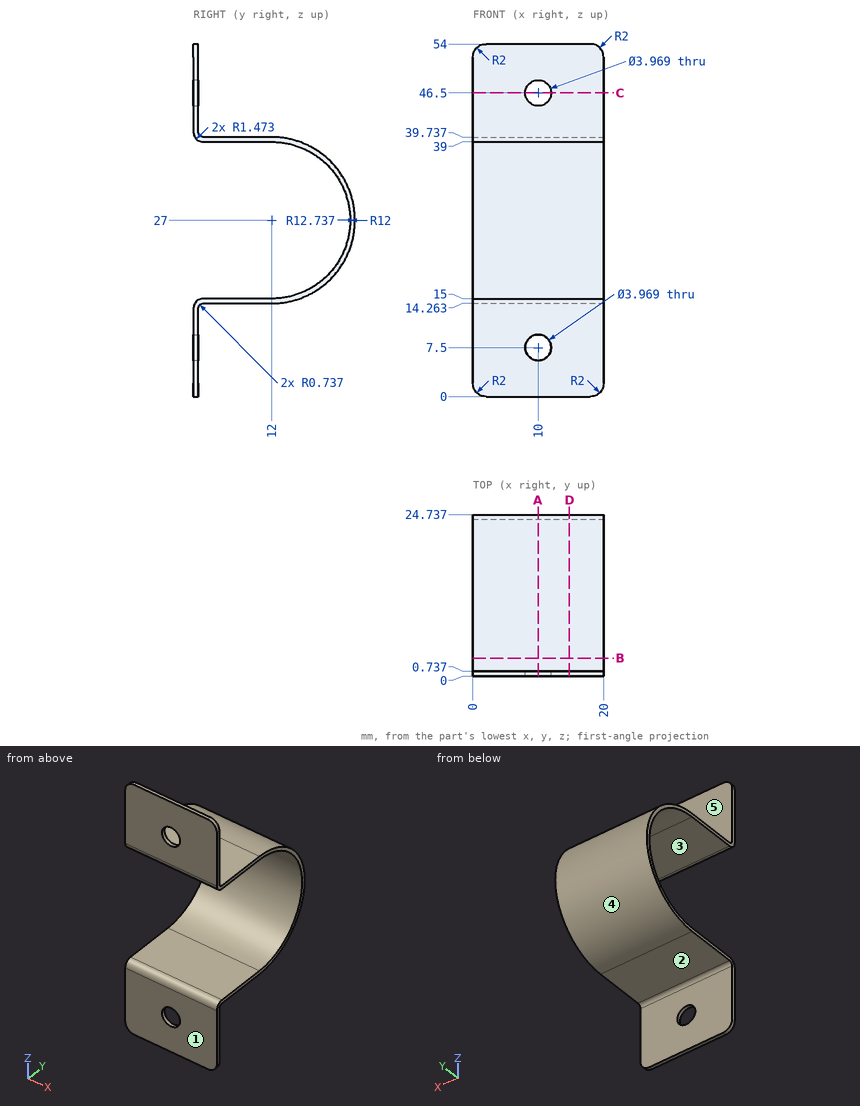
Drawing for the job (mm, zero at the part's lowest x, y, z). A direction names the side the tool comes from. Round coordinates to 2 decimals unless told otherwise and drop trailing zeros. Loops run counter-clockwise (first coordinate to the right, second up) from the corner with the lowest first, then second, coordinate; pieces in that order, holes last. Notation, with made-up numbers: (-8, 71.25) - (50, 71.25) arc R6 cw to (50, 77.25) - close; hole circle Ø10 at (85.5, 62.25). An arc over 180 degrees is marked (long way). Write each question's results on one line, items separated by ' | '.
(1) Saw through at C-C, the plane z = 46.5. List the corners of the cut face in (x, y) (1 decimal), then the cut area to 3 significant figures.
Answer below:
outline: (0, 0) - (8, 0) - (8, 0.7) - (0, 0.7) - close; (12, 0) - (20, 0) - (20, 0.7) - (12, 0.7) - close | area: 11.8 mm^2
(2) Saw through at D-D, the plane x = 14.75. List the corners of the cut face in (y, z).
Answer below:
outline: (0, 0) - (0.74, 0) - (0.74, 13.53) arc R0.74 cw to (1.47, 14.26) - (12, 14.26) arc R12.74 ccw to (12, 39.74) - (1.47, 39.74) arc R0.74 cw to (0.74, 40.47) - (0.74, 54) - (0, 54) - (0, 40.47) arc R1.47 ccw to (1.47, 39) - (12, 39) arc R12 cw to (12, 15) - (1.47, 15) arc R1.47 ccw to (0, 13.53) - close
(3) Pin check, flat tips, straight feed: pin 1 (5 mm diameter, centred on x = 10, z = 46.5, fed in from +Y); pin 2 (8.5 mm diameter, centred on x = 10, y = 9, fed in from +Z); pin 3 (6 mm diameter, centred on x = 5, y = 11, fed in from -Z). Stop position of each tip, or through.
Answer below:
pin 1: stops at y = 0.74 | pin 2: stops at z = 39.74 | pin 3: stops at z = 14.26
(4) Wall check: L1, parallel to X at y = 0.2, z = 7.5 (1 decimal); L2, parallel to Z at x = 11, y = 8.5; L3, parallel to Y at x = 8.25, z = 9.5. Give the ranges that are in metal, low to high.
Answer below:
L1: x = 0 to 8, 12 to 20 | L2: z = 14.26 to 15, 39 to 39.74 | L3: y = 0 to 0.74
(5) 3-axis set-ups, long thin cutter, end or side, ignore diameter. For the marked faces 1, 2, 3, 4 and 5: which of +Z, -Z, +X, -X, +Y, -Y reach the whole face in a straight line?
Answer below:
face 1: +Z, -Z, +X, -X, -Y | face 2: -Z, +X, -X, +Y | face 3: +X, -X, -Y | face 4: +X, -X, +Y | face 5: +Z, +X, -X, +Y
(6) Saw through at B-B, the plane y = 2.75. List the corners of the cut face in (x, z).
Answer below:
outline: (0, 14.26) - (20, 14.26) - (20, 15) - (0, 15) - close; (0, 39) - (20, 39) - (20, 39.74) - (0, 39.74) - close
(7) Saw through at A-A, the plane x = 10. List the corners of the cut face in (y, z) (1 decimal).
Answer below:
outline: (0, 0) - (0.7, 0) - (0.7, 5.5) - (0, 5.5) - close; (0, 9.5) - (0.7, 9.5) - (0.7, 13.5) arc R0.7 cw to (1.5, 14.3) - (12, 14.3) arc R12.7 ccw to (12, 39.7) - (1.5, 39.7) arc R0.7 cw to (0.7, 40.5) - (0.7, 44.5) - (0, 44.5) - (0, 40.5) arc R1.5 ccw to (1.5, 39) - (12, 39) arc R12 cw to (12, 15) - (1.5, 15) arc R1.5 ccw to (0, 13.5) - close; (0, 48.5) - (0.7, 48.5) - (0.7, 54) - (0, 54) - close
